Verification items for the finished model (mm, model axes). A direction names the side the tool comes from. Round coordinates to 2 decimals unless told otherwise and drop trailing zeros. Loops run counter-clockwise (first coordinate to the right, second up) from the corner with the lowest first, then second, coordinate; pieces in that order, holes last. Notation, with made-up numbers: (15.25, -12) -> (19.25, -12) arc R23 cw to (19.25, 15) -> close; hole circle Ø10 at (48, 35.25). An arc over 180 degrees is marked (long way). Use CSV: the item, a comma, the result in double quotes. Start each with the question number.
```python
from build123d import *

# Parameters (mm, degrees)
F0_W     = 17.23101
F0_H     = 56.631804
F1_DEPTH = 27.886009
F2_W     = 10
F2_H     = 9.07563
F3_DEPTH = 25.4


with BuildPart() as f1:
    # F0 (on Front) → F1 (new body)
    with BuildSketch(Plane.XZ):
        with Locations((-8.615505, 28.315902)):
            Rectangle(F0_W, F0_H)
    extrude(amount=F1_DEPTH)

    # F2 (on face) → F3 (join)
    with BuildSketch(Plane.YZ):
        with Locations((-15.322338, 30.503517)):
            Rectangle(F2_W, F2_H)
    extrude(amount=F3_DEPTH)


solid = f1.part
```
Q1. Cross-section at A-A (y = -18). Record the boundary of the cut face in (x, z).
Q2. Cross-section at C-C (x = 21). Record the boundary of the cut face in (y, z), and give its area (3 significant figures).
Q3. Cross-section at B-B (z = 33.5). Record the boundary of the cut face in (x, y).
Q4. Cross-section at D-D (y = -23.25). Record the boundary of the cut face in (x, z), and give its area (3 significant figures).
Q5. Thickness scan on L1, parallel to X at y = -9.25, z = 23.5; L2, parallel to Z at x = 6.5, y = -11. Record the ranges inside material, lowest first. Write a range as from..to.
Q6. Tool access check on faces 1 (the face through (13, -10.322, 30)), 2 (the face through (-17.231, -14, 28)), 3 (the face through (13, -20.322, 30)), 4 (the face through (13, -15, 35.041)), 5 (the face through (13, -15, 25.966)). Record the directions out of +Z, -Z, +X, -X, +Y, -Y that give a thin tool (end or side, any length) a straight path to the whole face; none if there is none.
Q7. Depth check by flat-ended pin: pin 1 Ø10 at (x, z) = (10.5, 32.5) entering from -Y; pin 2 Ø5 at (x, y) = (16, -15.5) entering from -Z; pin 3 Ø12 at (x, y) = (11, -12) entering from +Z. Enter the tip coordinate at first touch or a pass-through.
Answer list:
1,outline,"(-17.23, 0) -> (0, 0) -> (0, 25.97) -> (25.4, 25.97) -> (25.4, 35.04) -> (0, 35.04) -> (0, 56.63) -> (-17.23, 56.63) -> close"
2,outline,"(-20.32, 25.97) -> (-10.32, 25.97) -> (-10.32, 35.04) -> (-20.32, 35.04) -> close"
2,area,"90.8 mm2"
3,outline,"(-17.23, -27.89) -> (0, -27.89) -> (0, -20.32) -> (25.4, -20.32) -> (25.4, -10.32) -> (0, -10.32) -> (0, 0) -> (-17.23, 0) -> close"
4,outline,"(-17.23, 0) -> (0, 0) -> (0, 56.63) -> (-17.23, 56.63) -> close"
4,area,"976 mm2"
5,L1,"x = -17.23..0"
5,L2,"z = 25.97..35.04"
6,face 1,"+Z, -Z, +X, +Y"
6,face 2,"+Z, -Z, -X, +Y, -Y"
6,face 3,"+Z, -Z, +X, -Y"
6,face 4,"+Z, +X, +Y, -Y"
6,face 5,"-Z, +X, +Y, -Y"
7,pin 1,"stops at y = -20.32"
7,pin 2,"stops at z = 25.97"
7,pin 3,"stops at z = 35.04"
